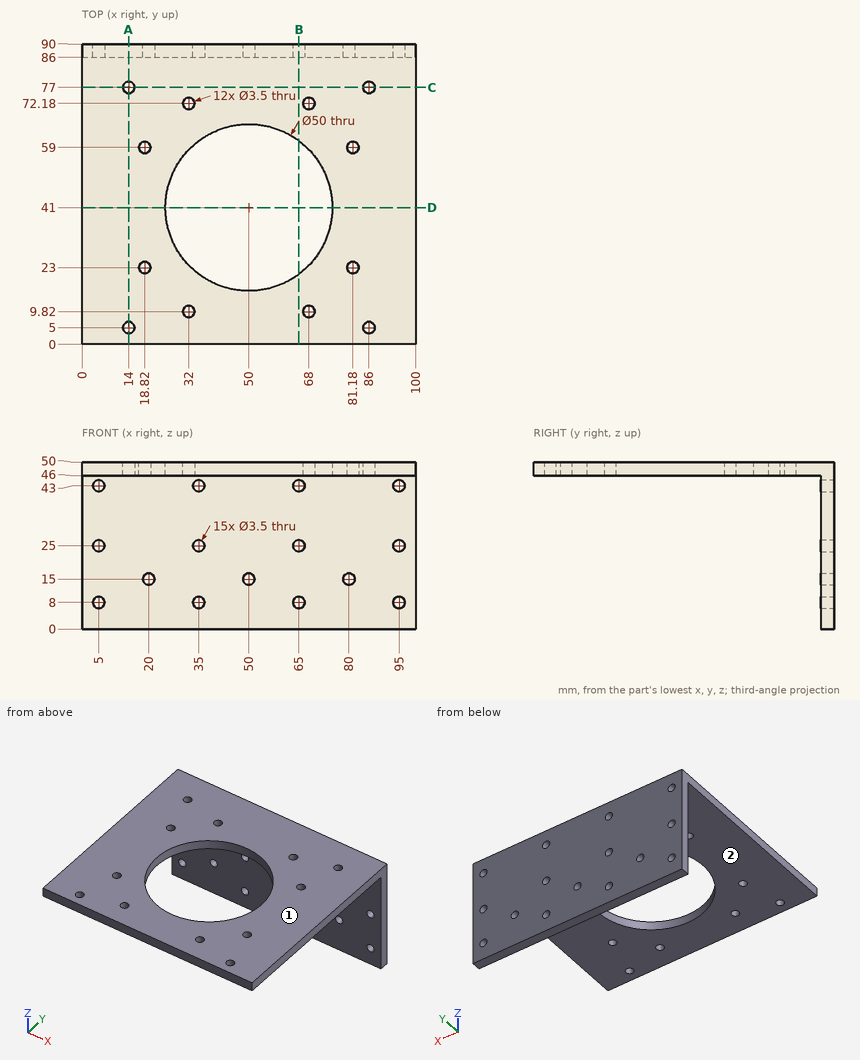
The drawing under review shows one solid part. Ordinate dimensions are in mm from its lowest x, y, z. A direction names the side the tool comes from. Coordinates: 2 decimals unless noted, no trailing zeros. Loops run counter-clockwise (first coordinate to the right, second up) from the corner with the lowest first, then second, coordinate; pieces in that order, holes last.
Item 1: Add section B-B (x = 65). Write out the cut boundary in (y, z), and give its area (3 significant figures).
Completed:
outline: (0, 46) - (21, 46) - (21, 50) - (0, 50) - close; (61, 46) - (86, 46) - (86, 44.75) - (90, 44.75) - (90, 50) - (61, 50) - close; (86, 0) - (90, 0) - (90, 6.25) - (86, 6.25) - close; (86, 9.75) - (90, 9.75) - (90, 23.25) - (86, 23.25) - close; (86, 26.75) - (90, 26.75) - (90, 41.25) - (86, 41.25) - close
area: 342 mm2
Item 2: Add section D-D (y = 41). Write out the cut boundary in (x, z).
Completed:
outline: (0, 46) - (25, 46) - (25, 50) - (0, 50) - close; (75, 46) - (100, 46) - (100, 50) - (75, 50) - close
Item 3: Add section A-A (x = 14). Write out the cut boundary in (y, z), and give its area (3 significant figures).
Completed:
outline: (0, 46) - (3.25, 46) - (3.25, 50) - (0, 50) - close; (6.75, 46) - (75.25, 46) - (75.25, 50) - (6.75, 50) - close; (78.75, 46) - (86, 46) - (86, 0) - (90, 0) - (90, 50) - (78.75, 50) - close
area: 516 mm2
Item 4: Clearance check with flat-ended pins moving along their axes: pin 1 (5.5 mm diameter, centred on x = 81.18, y = 23, fed in from +Z); pin 2 (3 mm diameter, centred on x = 68, y = 72.18, fed in from +Z); pin 3 (3 mm diameter, centred on x = 89, z = 32, fed in from -Y); pin 4 (4 mm diameter, centred on x = 86, y = 5, fed in from -Z). State where each tip first meets the part, or that it passes through.
Completed:
pin 1: stops at z = 50
pin 2: passes through
pin 3: stops at y = 86
pin 4: stops at z = 46
Item 5: Wall thickness on L1, parallel to X at y = 72.18, z = 47.2; L2, parallel to Y at x = 86, z = 49; L3, parallel to X at y = 87.8, z = 25: over which ranges is each line inside the solid? List them lowest first.
Completed:
L1: x = 0 to 30.25, 33.75 to 66.25, 69.75 to 100
L2: y = 0 to 3.25, 6.75 to 75.25, 78.75 to 90
L3: x = 0 to 3.25, 6.75 to 33.25, 36.75 to 63.25, 66.75 to 93.25, 96.75 to 100
Item 6: Add section C-C (y = 77). Write out the cut boundary in (x, z).
Completed:
outline: (0, 46) - (12.25, 46) - (12.25, 50) - (0, 50) - close; (15.75, 46) - (84.25, 46) - (84.25, 50) - (15.75, 50) - close; (87.75, 46) - (100, 46) - (100, 50) - (87.75, 50) - close
Item 7: For the marked faces 1 and 2, list the 3-axis set-ups (+Z, -Z, +X, -X, +Y, -Y) from which the entire face can be reached by the end or side of a thin tool; tool diameter is ignored.
Completed:
face 1: +Z, +X, -X, +Y, -Y
face 2: -Z, +X, -X, -Y
